Source: CAD feature listing. Evaluate the final solid. Frame: model axes, mm. Round coordinates to 2 decimals unless told otherwise and drop trailing zeros. Order: outer loops, then holes, each group sorted by start corner. A loop starts at its lowest first (then second) coordinate and runs counter-clockwise, first axis right, second up. Notation, with made-up numbers: (47.25, 44.5) -> (102.25, 44.5) arc R7 ccw to (102.25, 50.5) -> close; hole circle Ø8 at (82, -30.75). An arc over 180 degrees is marked (long way). Use a Markdown table: item, result. Add a question column.
```python
from build123d import *

# Parameters (mm, degrees)
SKETCH1_W            = 76
SKETCH1_H            = 64
BOSS_EXTRUDE1_DEPTH  = 8
M3_TAPPED_HOLE1_D    = 2.5
LPATTERN2_COUNT      = 2
LPATTERN2_PITCH      = 28
LPATTERN2_COUNT_DIR2 = 2
LPATTERN2_PITCH_DIR2 = 33
SKETCH5_R            = 2
CUT_EXTRUDE1_DEPTH   = 51.318982502
CHAMFER1_SIZE        = 1
SKETCH6_R            = 1.5
CUT_EXTRUDE2_DEPTH   = 10


with BuildPart() as part:
    # Sketch1 → Boss-Extrude1 (new body)
    with BuildSketch(Plane(origin=(0, 0, 0), x_dir=(1, 0, 0), z_dir=(0, 1, 0))):
        Rectangle(SKETCH1_W, SKETCH1_H)
    extrude(amount=BOSS_EXTRUDE1_DEPTH)

    # M3 Tapped Hole1 (through all)
    with Locations(Plane(origin=(0, 8, 0), x_dir=(1, 0, 0), z_dir=(0, 1, 0))):
        with Locations((-14, 26)):
            m3_tapped_hole1 = Hole(M3_TAPPED_HOLE1_D / 2)

    # LPattern2: M3 Tapped Hole1 2 × 2
    with Locations(*[(i * LPATTERN2_PITCH, 0, j * LPATTERN2_PITCH_DIR2) for i in range(LPATTERN2_COUNT) for j in range(LPATTERN2_COUNT_DIR2) if (i, j) != (0, 0)]):
        add(m3_tapped_hole1, mode=Mode.SUBTRACT)

    # Sketch5 → Cut-Extrude1 (cut, through all)
    with BuildSketch(Plane(origin=(0, 8, 0), x_dir=(1, 0, 0), z_dir=(0, 1, 0))):
        with Locations(Location((-33, 24, 0), (0, 0, 270))):
            Circle(SKETCH5_R)
        with Locations(Location((33, 24, 0), (0, 0, 270))):
            Circle(SKETCH5_R)
        with Locations(Location((0, -27, 0), (0, 0, 270))):
            Circle(SKETCH5_R)
    extrude(amount=-CUT_EXTRUDE1_DEPTH, mode=Mode.SUBTRACT)

    # Chamfer1
    chamfer1_edges = [part.edges().sort_by_distance(p)[0] for p in [
        (-38, 8, 0),
        (0, 8, 32),
        (38, 8, 0),
        (0, 8, -32),
    ]]
    chamfer(chamfer1_edges, length=CHAMFER1_SIZE)

    # Sketch6 → Cut-Extrude2 (cut)
    with BuildSketch(Plane(origin=(0, 8, 0), x_dir=(1, 0, 0), z_dir=(0, 1, 0))):
        with Locations(Location((32, -5.5, 0), (0, 0, 270))):
            Circle(SKETCH6_R)
        with Locations(Location((32, -23.5, 0), (0, 0, 270))):
            Circle(SKETCH6_R)
        with Locations(Location((-32, -23.5, 0), (0, 0, 270))):
            Circle(SKETCH6_R)
        with Locations(Location((-32, -5.5, 0), (0, 0, 270))):
            Circle(SKETCH6_R)
    extrude(amount=-CUT_EXTRUDE2_DEPTH, mode=Mode.SUBTRACT)


solid = part.part
```
1) Section A-A on z = 23.5. Output: boundary loops of the cut face in (x, y), then the cut area to 3 significant figures.
2) Section D-D on x = 0. Output: boundary loops of the cut face in (y, z), then the cut area to 3 significant figures.
3) Line query: probe 1 along Z at (x, y) = (14, 6); probe 2 along X at (y, z) = (3.5, 5.5); probe 3 along X at (y, z) = (0.5, 7.5). Output: solid intervals per line, ascending. Write a range as from..to.
4) Section C-C on y = 2. Count the separate pieces of the cut face and the enclosed holes in it, then the cut area to 3 significant figures.
5) Section B-B on x = 14. Output: boundary loops of the cut face in (y, z), then the cut area to 3 significant figures.
Conclusion:
| question | item | result |
|---|---|---|
| 1 | outline | (-38, 0) -> (-33.5, 0) -> (-33.5, 8) -> (-37, 8) -> (-38, 7) -> close; (-30.5, 0) -> (30.5, 0) -> (30.5, 8) -> (-30.5, 8) -> close; (33.5, 0) -> (38, 0) -> (38, 7) -> (37, 8) -> (33.5, 8) -> close |
| 1 | area | 559 mm^2 |
| 2 | outline | (0, -32) -> (7, -32) -> (8, -31) -> (8, 25) -> (0, 25) -> close; (0, 29) -> (8, 29) -> (8, 31) -> (7, 32) -> (0, 32) -> close |
| 2 | area | 479 mm^2 |
| 3 | probe 1 | z = -32..-27.25, -24.75..5.75, 8.25..32 |
| 3 | probe 2 | x = -38..-33.5, -30.5..30.5, 33.5..38 |
| 3 | probe 3 | x = -38..-15.15, -12.85..12.85, 15.15..38 |
| 4 | separate pieces | 1 |
| 4 | enclosed holes | 11 |
| 4 | area | 4,780 mm^2 |
| 5 | outline | (0, -32) -> (7, -32) -> (8, -31) -> (8, -27.25) -> (0, -27.25) -> close; (0, -24.75) -> (8, -24.75) -> (8, 5.75) -> (0, 5.75) -> close; (0, 8.25) -> (8, 8.25) -> (8, 31) -> (7, 32) -> (0, 32) -> close |
| 5 | area | 471 mm^2 |
